from build123d import *

# Parameters (mm, degrees)
SKETCH1_W                  = 340
SKETCH1_H                  = 550
BOSS_EXTRUDE1_DEPTH        = 1.3
F_5_0_5_DIAMETER_HOLE1_D   = 5
CONVERT_SOLID1_START       = -0.2
CONVERT_SOLID1_OUTLINE_W   = 340
CONVERT_SOLID1_OUTLINE_H   = 550
CONVERT_SOLID1_OUTLINE_R   = 2.5
CONVERT_SOLID1_DEPTH       = 0.2
SKETCHED_START             = -275
SKETCHED_BEND1_OUTLINE_W   = 1.5
SKETCHED_BEND1_OUTLINE_H   = 340
SKETCHED_BEND1_DEPTH       = 50.30822
SKETCHED_START_2           = -225
SKETCHED_BEND1_2_OUTLINE_W = 50.965708265
SKETCHED_BEND1_2_OUTLINE_H = 340
SKETCHED_BEND1_2_OUTLINE_R = 2.5
SKETCHED_BEND1_2_DEPTH     = 3
SKETCHED_START_3           = -171
SKETCHED_BEND1_3_DEPTH     = 342
F_5_0_5_DIAMETER_HOLE2_D   = 5
SKETCH10_2_R               = 12.5
CUT_EXTRUDE1_DEPTH         = 328.532670956
CUT_EXTRUDE3_DEPTH         = 328.32694619
CUT_EXTRUDE3_DEPTH_BACK    = 328.32694619
SKETCH1_4_R                = 1.5


with BuildPart() as part:
    # Sketch1 → Boss-Extrude1 (new body)
    with BuildSketch(Plane.YZ):
        Rectangle(SKETCH1_W, SKETCH1_H)
    extrude(amount=BOSS_EXTRUDE1_DEPTH)

    # Ø5.0 (5) Diameter Hole1 (through all)
    with Locations(Plane.YZ.offset(1.3)):
        with Locations((-157.3, -139.45), (-20, -139.45), (117.3, -139.45), (140, -250), (0, -250), (-140, -250)):
            Hole(F_5_0_5_DIAMETER_HOLE1_D / 2)

    # Convert-Solid1: read off the stored shape, not the designer's step
    # Convert-Solid1 outline → Convert-Solid1 (add)
    with BuildSketch(Plane.YZ.offset(CONVERT_SOLID1_START)):
        Rectangle(CONVERT_SOLID1_OUTLINE_W, CONVERT_SOLID1_OUTLINE_H)
        with Locations((-140, -250)):
            Circle(CONVERT_SOLID1_OUTLINE_R, mode=Mode.SUBTRACT)
        with Locations((-157.3, -139.45)):
            Circle(CONVERT_SOLID1_OUTLINE_R, mode=Mode.SUBTRACT)
        with Locations((-20, -139.45)):
            Circle(CONVERT_SOLID1_OUTLINE_R, mode=Mode.SUBTRACT)
        with Locations((0, -250)):
            Circle(CONVERT_SOLID1_OUTLINE_R, mode=Mode.SUBTRACT)
        with Locations((140, -250)):
            Circle(CONVERT_SOLID1_OUTLINE_R, mode=Mode.SUBTRACT)
        with Locations((117.3, -139.45)):
            Circle(CONVERT_SOLID1_OUTLINE_R, mode=Mode.SUBTRACT)
    extrude(amount=CONVERT_SOLID1_DEPTH)

    # Sketched Bend1: read off the stored shape, not the designer's step
    # Sketched Bend1 outline → Sketched Bend1 (cut)
    with BuildSketch(Plane.XY.offset(SKETCHED_START)):
        with Locations((0.55, 0)):
            Rectangle(SKETCHED_BEND1_OUTLINE_W, SKETCHED_BEND1_OUTLINE_H)
    extrude(amount=SKETCHED_BEND1_DEPTH, mode=Mode.SUBTRACT)

    # Sketched Bend1 2 outline → Sketched Bend1 2 (add)
    with BuildSketch(Plane.XY.offset(SKETCHED_START_2)):
        with Locations((-25.682854133, 0)):
            Rectangle(SKETCHED_BEND1_2_OUTLINE_W, SKETCHED_BEND1_2_OUTLINE_H)
        with Locations((-26.165708265, -140)):
            Circle(SKETCHED_BEND1_2_OUTLINE_R, mode=Mode.SUBTRACT)
        with Locations((-26.165708265, 0)):
            Circle(SKETCHED_BEND1_2_OUTLINE_R, mode=Mode.SUBTRACT)
        with Locations((-26.165708265, 140)):
            Circle(SKETCHED_BEND1_2_OUTLINE_R, mode=Mode.SUBTRACT)
    extrude(amount=SKETCHED_BEND1_2_DEPTH)

    # Sketched Bend1 3 outline → Sketched Bend1 3 (cut)
    with BuildSketch(Plane(origin=(0, 0, 0), x_dir=(1, 0, 0), z_dir=(0, 1, 0)).offset(SKETCHED_START_3)):
        with BuildLine():
            ThreePointArc((-0.2, 222), (-0.639339828, 223.060660172), (-1.7, 223.5))
            Line((-1.7, 223.5), (-51.165708265, 223.5))
            Line((-51.165708265, 223.5), (-51.165708265, 222))
            Line((-51.165708265, 222), (-0.2, 222))
        make_face()
        with BuildLine():
            Line((-0.2, 225), (-1.7, 225))
            ThreePointArc((-1.7, 225), (0.421320344, 224.121320344), (1.3, 222))
            Line((1.3, 222), (1.3, 224.69178))
            Line((1.3, 224.69178), (-0.2, 224.69178))
            Line((-0.2, 224.69178), (-0.2, 225))
        make_face()
    extrude(amount=SKETCHED_BEND1_3_DEPTH, mode=Mode.SUBTRACT)

    # Ø5.0 (5) Diameter Hole2 (through all)
    with Locations(Plane.YZ.offset(1.3)):
        with Locations((-28.578838325, 168.5), (0, 218), (28.578838325, 168.5)):
            Hole(F_5_0_5_DIAMETER_HOLE2_D / 2)

    # Sketch10<2> → Cut-Extrude1 (cut, through all)
    with BuildSketch(Plane.YZ.offset(1.3)):
        with Locations(Location((0, 185, 0), (0, 0, 270))):
            Circle(SKETCH10_2_R)
    extrude(amount=-CUT_EXTRUDE1_DEPTH, mode=Mode.SUBTRACT)

    # Sketch1<4> → Cut-Extrude3 (cut, two sides: drawn at the far end of the back side and taken through both)
    with BuildSketch(Plane.YZ.offset(-CUT_EXTRUDE3_DEPTH_BACK)):
        with Locations(Location((156.891480577, 262.3, 0), (0, 0, 270))):
            Circle(SKETCH1_4_R)
        with Locations(Location((132.789034574, 262.3, 0), (0, 0, 270))):
            Circle(SKETCH1_4_R)
    extrude(amount=CUT_EXTRUDE3_DEPTH + CUT_EXTRUDE3_DEPTH_BACK, mode=Mode.SUBTRACT)


solid = part.part
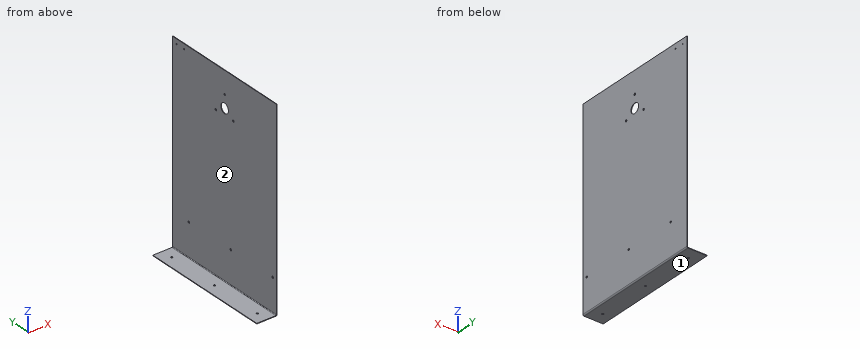
Could you check a few things on this model? Use its own coordinates, in mm. Face numbers are marked on the shaded views. A direction names the side the tool comes from. Give positions to 0.01 mm unless a question says otherwise; leave off trailing zeros. Order: outer loops, then holes, each group sorted by start corner. A loop starts at its lowest first (then second) coordinate and runs counter-clockwise, first axis right, second up.
Item 1: For the marked faces 1 and 2, which set-ups out of +Z, -Z, +X, -X, +Y, -Y let a thin tool reach every point of the face, with its end or its side?
Item 2: If we section it at A-A, the plane z = 185: Write out the boundary of the cut face in (x, y), plus the area to 4 significant figures.
Item 3: I need wall thicknesses on line 1 (Y direction, x = 0, z = -139); line 2 (Y direction, x = 0.25, z = 262.3); line 3 (X direction, y = 44.5, z = 147). Which ranges of each line are inside material? Lowest first, please.
Item 4: If we section it at D-D, the plane z = 4.5: Write out the boundary of the cut face in (x, y).
Item 5: If we section it at B-B, the plane y = 48.5: Write out the boundary of the cut face in (x, z).
Item 6: I'm going to push flat-ended pins straight in: pin 1 (6 mm diameter, centred on y = -157.3, z = -139.45, fed in from -X); pin 2 (1.5 mm diameter, centred on x = -14.5, y = -78.5, fed in from +Z). Where does each tip first touch, or does it pass through?
Item 7: If we section it at C-C, the plane x = -36.5: Write out the boundary of the cut face in (y, z), plus the area to 3 significant figures.
Values:
1. face 1: -Z, +X, -X, +Y, -Y
1. face 2: +Z, -X, +Y, -Y
2. outline: (-0.2, -170) - (1.3, -170) - (1.3, -12.5) - (-0.2, -12.5) - close; (-0.2, 12.5) - (1.3, 12.5) - (1.3, 170) - (-0.2, 170) - close
2. area: 472.5 mm2
3. line 1: y = -170 to -159.76, -154.84 to -22.46, -17.54 to 114.84, 119.76 to 170
3. line 2: y = -170 to 131.29, 134.29 to 155.39, 158.39 to 170
3. line 3: x = -0.2 to 1.3
4. outline: (-0.2, -170) - (1.3, -170) - (1.3, 170) - (-0.2, 170) - close
5. outline: (-51.17, -225) - (-1.7, -225) arc R3 ccw to (1.3, -222) - (1.3, 275) - (-0.2, 275) - (-0.2, -222) arc R1.5 cw to (-1.7, -223.5) - (-51.17, -223.5) - close
6. pin 1: stops at x = -0.2
6. pin 2: stops at z = -223.5
7. outline: (-170, -225) - (170, -225) - (170, -223.5) - (-170, -223.5) - close
7. area: 510 mm2
